Study the drawing (mm; zero at the part's minimum x, y, z) and answer. A direction names the side the tool comes from. Coordinates: 2 decimals unless noted, no trailing zeros. Loops run counter-clockwise (first coordinate to the right, second up) from the corner with the lowest first, then second, coordinate; pieces in that order, holes last. Notation, with made-up numbers: (71.5, 69.25) - (103.5, 69.25) arc R31 cw to (103.5, 104.25) - close; hole circle Ø1 at (16.5, 86.5). An arc over 180 degrees is marked (long way). Use one line per item in the form item = value.
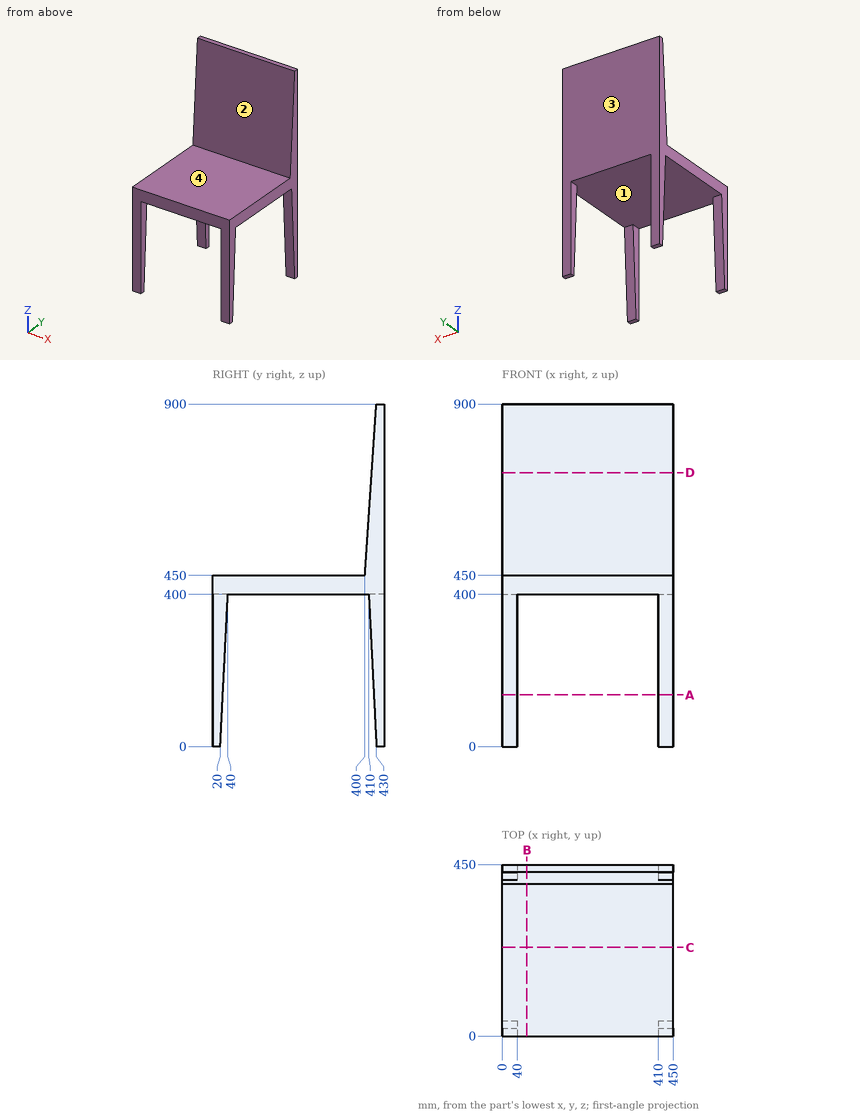
Item 1: Which of the six approach directions +Z, -Z, +X, -X, +Y, -Y give full straight-line access (tool end or side, diameter ignored) to the marked faces 3 and 4?
Results below:
face_3 = +Z, -Z, +X, -X, +Y
face_4 = +Z, +X, -X, -Y
Item 2: Each of these flat-tipped pins is pushed along its axis until it touches: P1, Ø8, axis at x = 183, y = 137, coming from the +Z side; P2, Ø12, axis at x = 261, y = 45.5, coming from the -Z side. Where does it stop, or does it pass through?
Results below:
P1 = 450
P2 = 400
Item 3: The part is cut by section B-B on x = 65. Give the vertices of the cut face in (y, z), plus the area to 4 significant figures.
Results below:
outline = (0, 400) - (450, 400) - (450, 900) - (430, 900) - (400, 450) - (0, 450) - close
area = 38,250 mm²
Item 4: Find the intervals of material crossed by L1, parallel to Y at x = 320, z = 599; L2, parallel to Z at x = 184, y = 153; L3, parallel to Z at x = 419, y = 19.5, in increasing order.
Results below:
L1 = 409.93 to 450
L2 = 400 to 450
L3 = 0 to 450
Item 5: The part is cut by section D-D on z = 720. Give the vertices of the cut face in (x, y).
Results below:
outline = (0, 418) - (450, 418) - (450, 450) - (0, 450) - close
Item 6: The part is cut by section C-C on y = 233. Give the vertices of the cut face in (x, z), plus the area to 3 significant figures.
Results below:
outline = (0, 400) - (450, 400) - (450, 450) - (0, 450) - close
area = 22,500 mm²
Item 7: For a pull along X with two mould halves and no side action, classify the marked faces 1 and 2 as +X half, -X half, draft (parallel to the pull), parting line (faces both ways), or undercut.
Results below:
face_1 = undercut
face_2 = draft
Item 8: The part is cut by section A-A on z = 136. Give the vertices of the cut face in (x, y), plus the area to 3 significant figures.
Results below:
outline = (0, 0) - (40, 0) - (40, 26.8) - (0, 26.8) - close; (0, 423.2) - (40, 423.2) - (40, 450) - (0, 450) - close; (410, 0) - (450, 0) - (450, 26.8) - (410, 26.8) - close; (410, 423.2) - (450, 423.2) - (450, 450) - (410, 450) - close
area = 4,290 mm²
